Geometry check sheet. Reference: the model listing, model coordinates, mm. A direction names the side the tool comes from. Give positions to 0.01 mm unless a question says otherwise; leave off trailing zeros. Loops run counter-clockwise (first coordinate to the right, second up) from the corner with the lowest first, then second, coordinate; pieces in that order, holes last. Notation, with made-up numbers: (8, 84.25) -> (52, 84.25) arc R18 ccw to (52, 93.25) -> close; hole circle Ø2 at (70, 55). An arc over 180 degrees is marked (long way). Write item = value, one per line.
```python
from build123d import *

# Parameters (mm, degrees)
SKETCH1_R            = 5.5
SKETCH1_R_2          = 1.75
BOSS_EXTRUDE1_DEPTH  = 28.5
CUT_EXTRUDE1_DEPTH   = 74.164092839
SKETCH3_W            = 9
SKETCH3_H            = 25
CUT_EXTRUDE2_DEPTH   = 28
SKETCH4_W            = 16
SKETCH4_H            = 14.8
CUT_EXTRUDE3_DEPTH   = 26.000210526
M4_CLEARANCE_HOLE1_D = 4.5
SKETCH6_R            = 3.994459126
SKETCH6_R_2          = 4.1
CUT_EXTRUDE4_DEPTH   = 30
SKETCH7_W            = 9
SKETCH7_H            = 15
CUT_EXTRUDE5_DEPTH   = 59.773195259


with BuildPart() as part:
    # Sketch1 → Boss-Extrude1 (new, symmetric)
    with BuildSketch(Plane(origin=(0, 0, 0), x_dir=(1, 0, 0), z_dir=(0, 1, 0))):
        with BuildLine():
            Line((0, 0), (64.191, 0))
            Line((64.191, 0), (64.191, -16))
            Line((64.191, -16), (44.191, -16))
            Line((44.191, -16), (44.191, -25.5))
            ThreePointArc((44.191, -25.5), (41.583024376, -32.038348415), (35.191, -34.986832981))
            Line((35.191, -34.986832981), (35.191, -32.983314774))
            ThreePointArc((35.191, -32.983314774), (34.691, -18), (34.191, -32.983314774))
            Line((34.191, -32.983314774), (34.191, -34.986832981))
            ThreePointArc((34.191, -34.986832981), (29.296680203, -33.319930558), (26.000210526, -29.336688458))
            ThreePointArc((26.000210526, -29.336688458), (13.741809885, -36.325925267), (4.691, -25.5))
            Line((4.691, -25.5), (4.691, -16))
            Line((4.691, -16), (0, -16))
            Line((0, -16), (0, 0))
        make_face()
        with Locations(Location((15.691, -25.5, 0), (0, 0, 90))):
            Circle(SKETCH1_R, mode=Mode.SUBTRACT)
        with Locations(Location((10.765708197, -31.804086029, 0), (0, 0, 90))):
            Circle(SKETCH1_R_2, mode=Mode.SUBTRACT)
        with Locations(Location((9.386913971, -20.574708197, 0), (0, 0, 90))):
            Circle(SKETCH1_R_2, mode=Mode.SUBTRACT)
        with Locations(Location((20.616291803, -19.195913971, 0), (0, 0, 90))):
            Circle(SKETCH1_R_2, mode=Mode.SUBTRACT)
        with Locations(Location((21.995086029, -30.425291803, 0), (0, 0, 90))):
            Circle(SKETCH1_R_2, mode=Mode.SUBTRACT)
    extrude(amount=BOSS_EXTRUDE1_DEPTH, both=True)

    # Sketch2 → Cut-Extrude1 (cut, through all)
    with BuildSketch(Plane.XY.offset(16)):
        Polygon((4.691, 18.5), (26.000210526, 18.5), (26.000210526, -19.5), (44.191, -19.5), (44.191, -28.5), (4.691, -28.5), align=None)
    extrude(amount=CUT_EXTRUDE1_DEPTH, mode=Mode.SUBTRACT)

    # Sketch3 → Cut-Extrude2 (cut)
    with BuildSketch(Plane.ZY):
        with Locations((8, 0)):
            Rectangle(SKETCH3_W, SKETCH3_H)
    extrude(amount=-CUT_EXTRUDE2_DEPTH, mode=Mode.SUBTRACT)

    # Sketch4 → Cut-Extrude3 (cut)
    with BuildSketch(Plane.ZY):
        with Locations((8, 0)):
            Rectangle(SKETCH4_W, SKETCH4_H)
    extrude(amount=-CUT_EXTRUDE3_DEPTH, mode=Mode.SUBTRACT)

    # M4 Clearance Hole1 (through all)
    with Locations(Plane(origin=(54.191, 0, 16), x_dir=(1, 0, 0), z_dir=(0, 0, 1))):
        with Locations((0, 0)):
            Hole(M4_CLEARANCE_HOLE1_D / 2)

    # Sketch6 → Cut-Extrude4 (cut)
    with BuildSketch(Plane.ZY):
        with Locations((8, -22.5)):
            Circle(SKETCH6_R)
        with Locations((8, 22.5)):
            Circle(SKETCH6_R_2)
    extrude(amount=-CUT_EXTRUDE4_DEPTH, mode=Mode.SUBTRACT)

    # Sketch7 → Cut-Extrude5 (cut, through all)
    with BuildSketch(Plane.ZY.offset(-28)):
        with Locations((8, 0)):
            Rectangle(SKETCH7_W, SKETCH7_H)
    extrude(amount=-CUT_EXTRUDE5_DEPTH, mode=Mode.SUBTRACT)


solid = part.part
```
Item 1: Section check B-B, the plane x = 33. Record the cut outline in (y, z), plus the area to 3 significant figures.
Answer:
outline = (-28.5, 0) -> (28.5, 0) -> (28.5, 18.19) -> (-19.5, 18.19) -> (-19.5, 16) -> (-28.5, 16) -> close; (-19.5, 32.81) -> (28.5, 32.81) -> (28.5, 34.85) -> (-19.5, 34.85) -> close; hole (-7.5, 3.5) -> (7.5, 3.5) -> (7.5, 12.5) -> (-7.5, 12.5) -> close
area = 980 mm^2
Item 2: Gauge pin test, flat ends, axial feed: pin 1 (6 mm diameter, centred on y = -5, z = 13.5, fed in from -X); pin 2 (1 mm diameter, centred on y = -3.5, z = 2, fed in from -X); pin 3 (3 mm diameter, centred on x = 29.5, z = 31.5, fed in from -Y); pin 4 (8 mm diameter, centred on y = -13.5, z = 30.5, fed in from +X). Record the tip position at first contact, or that the pin passes through.
Answer:
pin_1 = 0
pin_2 = 26
pin_3 = -19.5
pin_4 = 44.14
Item 3: Section check D-D, the plane z = 14.5. Record the cut outline in (x, y), plus the area to 3 significant figures.
Answer:
outline = (0, -28.5) -> (64.19, -28.5) -> (64.19, 28.5) -> (0, 28.5) -> (0, 7.4) -> (26, 7.4) -> (26, -7.4) -> (0, -7.4) -> close; hole circle Ø4.5 at (54.19, 0)
area = 3,260 mm^2
Item 4: Section check C-C, the plane z = 8. Record the cut outline in (x, y), plus the area to 3 significant figures.
Answer:
outline = (0, -28.5) -> (64.19, -28.5) -> (64.19, -7.5) -> (28, -7.5) -> (28, -12.5) -> (0, -12.5) -> (0, -18.51) -> (30, -18.51) -> (30, -26.49) -> (0, -26.49) -> close; (0, 12.5) -> (28, 12.5) -> (28, 7.5) -> (64.19, 7.5) -> (64.19, 28.5) -> (0, 28.5) -> (0, 26.6) -> (30, 26.6) -> (30, 18.4) -> (0, 18.4) -> close
area = 1,930 mm^2
Item 5: Tool access check on faces 4 (the flat face through (39, -19.5, 19)), 5 (the flat face through (34.191, 5, 34)), 6 (the flat face through (44.191, 5, 21)), 7 (the flat face through (46, 7.5, 8)), 8 (the flat face through (14, 12.5, 8)). Record the directions out of +Z, -Z, +X, -X, +Y, -Y that give a thin tool (end or side, any length) a straight path to the whole face; none if there is none.
Answer:
face_4 = +Z, +X, -X, -Y
face_5 = +Z, +Y, -Y
face_6 = +Z, +X, +Y, -Y
face_7 = +X, -X
face_8 = -X
Item 6: Draft check along Y on faces 1 (the cylindrical face through (14.8, -19.1, 10.1)), 2 (the flat face through (33, -28.5, 8)), 3 (the flat face through (33, 28.5, 14)). Enter one of: +Y half, -Y half, draft (parallel to the pull), parting line (faces both ways), or undercut.
Answer:
face_1 = undercut
face_2 = -Y half
face_3 = +Y half
Item 7: Thickness scan on L1, parallel to X at y = 22.5, z = 25.5; L2, parallel to Z at x = 15.5, y = 21; L3, parallel to X at y = 22.5, z = 28. Record the ranges inside material, lowest first. Write a range as [from, to].
Answer:
L1 = [4.69, 10.19], [21.19, 27.19], [42.19, 44.19]
L2 = [0, 4.18], [11.82, 20], [31, 36.5]
L3 = [4.98, 10.79], [20.59, 27.62], [41.76, 43.86]
Item 8: Section check A-A, the plane y = 0. Record the cut outline in (x, z).
Answer:
outline = (26, 0) -> (51.94, 0) -> (51.94, 3.5) -> (26, 3.5) -> close; (26, 12.5) -> (51.94, 12.5) -> (51.94, 16) -> (44.19, 16) -> (44.19, 25.5) arc R9.5 ccw to (35.19, 34.99) -> (35.19, 32.98) arc R7.5 cw (long way) to (34.19, 32.98) -> (34.19, 34.99) arc R9.5 ccw to (26, 29.34) -> close; (56.44, 0) -> (64.19, 0) -> (64.19, 3.5) -> (56.44, 3.5) -> close; (56.44, 12.5) -> (64.19, 12.5) -> (64.19, 16) -> (56.44, 16) -> close
